Here's how the part is built. I have some questions about the finished solid (model axes, mm). A direction names the side the tool comes from. Give positions to 0.01 mm unless a question says otherwise; leave off trailing zeros. Loops run counter-clockwise (first coordinate to the right, second up) from the corner with the lowest first, then second, coordinate; pieces in that order, holes last. Notation, with made-up numbers: (-24, 74) - (30, 74) arc R29 ccw to (30, 103) - close; hole circle Ø9 at (72.25, 46.25). An arc over 180 degrees is marked (long way). Return JSON: item names as keys, results as strings. Group by question number.
(1) If we section it at D-D (x = -9.5): State how many separate pieces and enclosed holes the cut face has, then the cut area to 3 significant figures.
(2) I need wall thicknesses on probe 1 along X at (y, z) = (0.5, -2); probe 2 along Y at (x, z) = (-11.5, -0.5); probe 3 along Y at (x, z) = (11.5, 2.25). Which ranges of each line are inside material? Lowest first, please. Write a range as [from, to].
(3) If we mould it in two halves opening along Y, with no side actions, what happens to faces 4 (the flat face through (4, -11, 3.5)), 5 (the cylindrical face through (-13.887, -10.648, 0.049)), 6 (the cylindrical face through (4.22, 10.16, 0.24))? For each: released by +Y, released by -Y, zero draft, split by the parting line, or undercut.
(4) On a 3-axis mill with a long thin cutter (end or side, diameter ignored), from which of +Z, -Z, +X, -X, +Y, -Y can I reach the whole of each face in a straight line? I mean faces 1 (the cylindrical face through (-13, -4, 0)), 2 (the flat face through (4, -11, -3.5)), 3 (the cylindrical face through (10.167, 4.199, 0.243)). Say none if no direction works.
(5) For P1, Ø2, axis at x = -13, z = 1.5, coming from the -Y side; P2, Ø3, axis at x = -12.5, z = 0.5, coming from the -Y side; P3, Ø2, axis at x = -3, z = 1, coming from the +Y side, each with a flat end and sliding along its axis, tell me the tip position at first contact or that it passes through.
(6) If we section it at A-A (y = 0): Please give me the cut outline in (x, z), then the cut area to 3 significant figures.
```python
from build123d import *

# Parameters (mm, degrees)
SKETCH1_R           = 17.5
SKETCH1_R_2         = 11
BOSS_EXTRUDE1_DEPTH = 3.5
SKETCH4_R           = 4
CUT_EXTRUDE1_DEPTH  = 6.2
CIRPATTERN1_COUNT   = 8


with BuildPart() as part:
    # Sketch1 → Boss-Extrude1 (new body, symmetric)
    with BuildSketch(Plane.XY):
        Circle(SKETCH1_R)
        Circle(SKETCH1_R_2, mode=Mode.SUBTRACT)
    extrude(amount=BOSS_EXTRUDE1_DEPTH, both=True)

    # Sketch4 → Cut-Extrude1 (cut)
    with BuildSketch(Plane(origin=(-10.162674858, 0, 0), x_dir=(0, 0, -1), z_dir=(1, 0, 0))):
        Circle(SKETCH4_R)
    cut_extrude1 = extrude(amount=-CUT_EXTRUDE1_DEPTH, mode=Mode.SUBTRACT)

    # CirPattern1: Cut-Extrude1 ×8 about axis
    cirpattern1_axis = Axis((0, 0, 0), (0, 0, 1))
    for i in range(1, CIRPATTERN1_COUNT):
        add(cut_extrude1.rotate(cirpattern1_axis, i * 360 / CIRPATTERN1_COUNT), mode=Mode.SUBTRACT)


solid = part.part
```
Values:
{
 "1": {"separate pieces": "6", "enclosed holes": "0", "area": "18.1 mm2"},
 "2": {"probe 1": "[-17.49, -16.36], [16.36, 17.49]", "probe 2": "[-13.19, -11.64], [-5.89, -3.97], [3.97, 5.89], [11.64, 13.19]", "probe 3": "[-13.19, -11.64], [-6.82, -3.31], [3.31, 6.82], [11.64, 13.19]"},
 "3": {"face 4": "zero draft", "face 5": "split by the parting line", "face 6": "undercut"},
 "4": {"face 1": "none", "face 2": "-Z, +X, -X, +Y, -Y", "face 3": "+Z, -Z"},
 "5": {"P1": "y = -12.74", "P2": "y = -13.61", "P3": "y = 17.39"},
 "6": {"outline": "(-17.5, -3.5) - (-16.36, -3.5) - (-16.36, 3.5) - (-17.5, 3.5) - close; (16.36, -3.5) - (17.5, -3.5) - (17.5, 3.5) - (16.36, 3.5) - close", "area": "15.9 mm2"}
}
